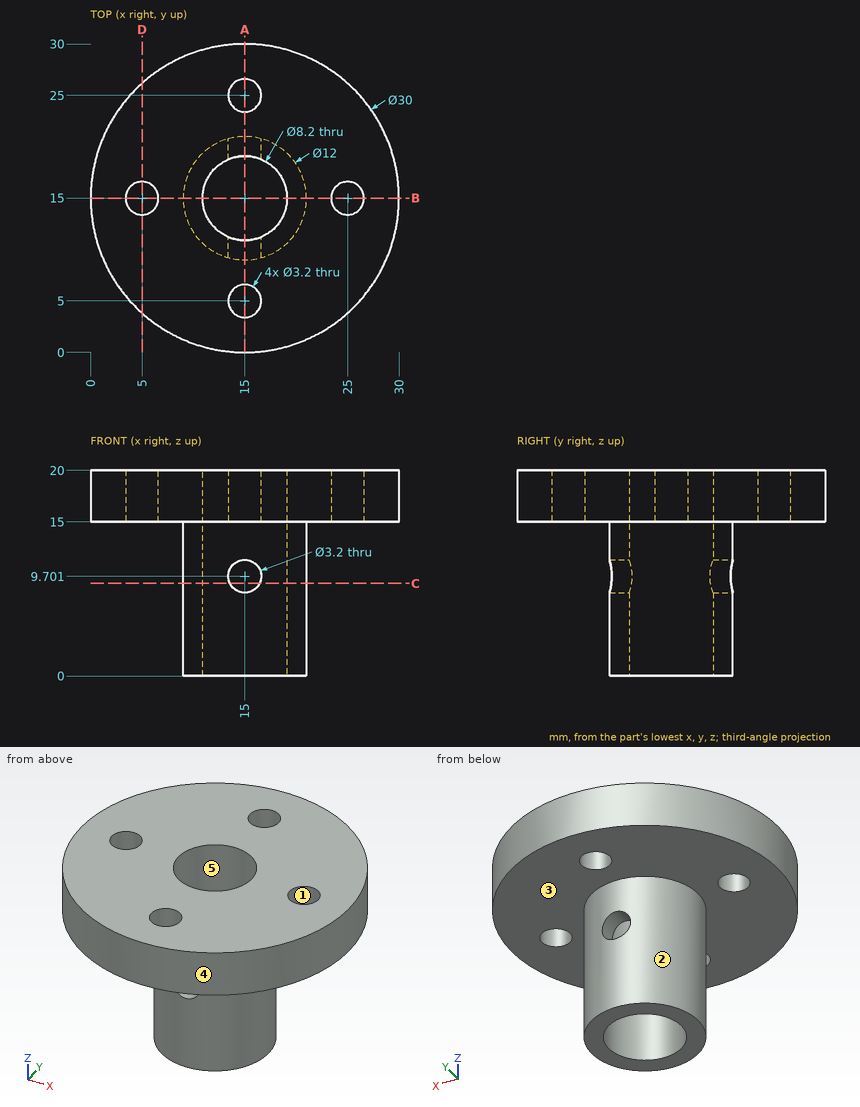
Print and shaded views of the part. All mm, measured from the part's lowest x, y and z. A direction names the side the tool comes from. Round coordinates to 2 decimals unless told otherwise and drop trailing zeros. Write each loop counter-clockwise with the first axis right and the second up, starting at its lowest first coordinate (ties: lowest second). Pieces come first, ordered by that corner, then holes.
Item 1: Which spindle directions (+Z, -Z, +X, -X, +Y, -Y) get a long thin tool onto all of the face, cutting with end or side? Do the marked faces 1 and 2. Say none if no direction does.
Results:
face 1: +Z, -Z
face 2: -Z
Item 2: Probe L1, parallel to Y at x = 15, z = 17; L2, parallel to Y at x = 16.25, z = 17.75 (1 decimal); L3, parallel to Z at x = 4, y = 11.25. List the from-to ranges inside material, lowest first.
Results:
L1: y = 0 to 3.4, 6.6 to 10.9, 19.1 to 23.4, 26.6 to 30
L2: y = 0.1 to 4, 6 to 11.1, 18.9 to 24, 26 to 29.9
L3: z = 15 to 20
Item 3: Cut at D-D, the plane x = 5. Give the cut face in (y, z).
Results:
outline: (3.82, 15) - (13.4, 15) - (13.4, 20) - (3.82, 20) - close; (16.6, 15) - (26.18, 15) - (26.18, 20) - (16.6, 20) - close
Item 4: Cut at A-A, the plane x = 15. Give the cut face in (y, z).
Results:
outline: (0, 15) - (3.4, 15) - (3.4, 20) - (0, 20) - close; (6.6, 15) - (9, 15) - (9, 11.3) - (10.9, 11.3) - (10.9, 20) - (6.6, 20) - close; (9, 0) - (10.9, 0) - (10.9, 8.1) - (9, 8.1) - close; (19.1, 0) - (21, 0) - (21, 8.1) - (19.1, 8.1) - close; (19.1, 11.3) - (21, 11.3) - (21, 15) - (23.4, 15) - (23.4, 20) - (19.1, 20) - close; (26.6, 15) - (30, 15) - (30, 20) - (26.6, 20) - close
Item 5: Drop flat-ended pins along their axis: pin 1 Ø5 at (x, y) = (7, 9.5) entering from -Z; pin 2 Ø4 at (x, y) = (5, 15) entering from +Z; pin 3 Ø3 at (y, z) = (11.5, 7.5) entering from -X; pin 4 Ø10 at (y, z) = (17.5, 10.5) entering from -X. Give the stop position or say it passes through.
Results:
pin 1: stops at z = 15
pin 2: stops at z = 20
pin 3: stops at x = 9.34
pin 4: stops at x = 0
Item 6: Cut at B-B, the plane y = 15. Give the cut face in (x, z), plus the area to 3 significant figures.
Results:
outline: (0, 15) - (3.4, 15) - (3.4, 20) - (0, 20) - close; (6.6, 15) - (9, 15) - (9, 0) - (10.9, 0) - (10.9, 20) - (6.6, 20) - close; (19.1, 0) - (21, 0) - (21, 15) - (23.4, 15) - (23.4, 20) - (19.1, 20) - close; (26.6, 15) - (30, 15) - (30, 20) - (26.6, 20) - close
area: 134 mm2
Item 7: Two-plate mould, pull along X, no slides. Class the marked faces 3, 4 and 5: +X half, -X half, draft (parallel to the pull), parting line (faces both ways), or undercut.
Results:
face 3: draft
face 4: parting line
face 5: undercut
Item 8: Cut at C-C, the plane z = 9. Give the cut face in (x, y) (1 decimal).
Results:
outline: (13.6, 9.2) - (13.6, 11.2) arc R4.1 cw to (13.6, 18.8) - (13.6, 20.8) arc R6 ccw to start; (16.4, 9.2) arc R6 ccw to (16.4, 20.8) - (16.4, 18.8) arc R4.1 cw to (16.4, 11.2) - close
